from build123d import *

# Parameters (mm, degrees)
PROFILE_SKETCH_W         = 25
PROFILE_SKETCH_H         = 10.810660172
THICKNESS_EXTRUDE_DEPTH  = 2
FILLETS_R                = 6
CONNECTION_CHAMFER_SIZE  = 0.75
CONNECTION_CHAMFER_SIZE2 = 1.810660172


with BuildPart() as part:
    # Profile Sketch → Thickness Extrude (new body)
    with BuildSketch(Plane(origin=(0, 0, 0), x_dir=(1, 0, 0), z_dir=(0, 1, 0))):
        with Locations((12.5, 5.405330086)):
            Rectangle(PROFILE_SKETCH_W, PROFILE_SKETCH_H)
    extrude(amount=THICKNESS_EXTRUDE_DEPTH)

    # Fillets
    fillets_edges = [part.edges().sort_by_distance(p)[0] for p in [
        (0, 1, -10.810660172),
        (25, 1, -10.810660172),
    ]]
    fillet(fillets_edges, radius=FILLETS_R)

    # Connection Chamfer
    connection_chamfer_edges = [part.edges().sort_by_distance(p)[0] for p in [
        (12.5, 0, 0),
        (12.5, 2, 0),
    ]]
    connection_chamfer_side = [part.faces().sort_by_distance(p)[0] for p in [
        (12.5, 1, 0),
    ]]
    chamfer(connection_chamfer_edges, length=CONNECTION_CHAMFER_SIZE, length2=CONNECTION_CHAMFER_SIZE2, reference=connection_chamfer_side[0])


solid = part.part
Could you check a few things on this model? Use its own coordinates, in mm. Give positions to 0.01 mm unless a question says otherwise; leave off trailing zeros. Write each loop counter-clockwise with the first axis right and the second up, starting at its lowest first coordinate (ties: lowest second). Pieces come first, ordered by that corner, then holes. Notation, with made-up numbers: (-6, 70.25) -> (18, 70.25) arc R28 ccw to (18, 89.25) -> close; hole circle Ø7 at (66.25, 24.25). An arc over 180 degrees is marked (long way). Answer as a JSON object with one key per item and string values.
Q1. Suppose I cut it at A-A on x = 7.25. Write out the boundary of the cut face in (y, z), then the cut area to 3 significant figures.
Taken from the geometry:
{"outline": "(0, -10.81) -> (2, -10.81) -> (2, -1.81) -> (1.25, 0) -> (0.75, 0) -> (0, -1.81) -> close", "area": "20.3 mm²"}
Q2. We'd pull the mould along Z, two halves only. Please class faces 1 (the flat face through (25, 1, -3)), 2 (the flat face through (12.32, 0.37, -0.92)), 3 (the cylindrical face through (23.289, 1.014, -9.006)): released by +Z, released by -Z, zero draft, split by the parting line, or undercut.
Taken from the geometry:
{"face 1": "zero draft", "face 2": "released by +Z", "face 3": "released by -Z"}
Q3. Suppose I cut it at C-C on z = -8.75. Write out the boundary of the cut face in (x, y), then the cut area to 3 significant figures.
Taken from the geometry:
{"outline": "(1.47, 0) -> (23.53, 0) -> (23.53, 2) -> (1.47, 2) -> close", "area": "44.1 mm²"}
Q4. Will this pin go through, and if not, where does the flat tip stop? pin 1 Ø1 at (y, z) = (0.5, -5.5) entering from -X.
Taken from the geometry:
{"pin 1": "stops at x = 0"}
Q5. Please list where these lines run through material, in increasing order: L1, parallel to X at y = 1.85, z = -6.5; L2, parallel to Z at x = 6, y = 1.45; L3, parallel to X at y = 0.5, z = -7.
Taken from the geometry:
{"L1": "x = 0.24 to 24.76", "L2": "z = -10.81 to -0.48", "L3": "x = 0.41 to 24.59"}
Q6. Suppose I cut it at B-B on y = 1.5. Write out the boundary of the cut face in (x, z), then the cut area to 3 significant figures.
Taken from the geometry:
{"outline": "(0, -4.81) arc R6 ccw to (6, -10.81) -> (19, -10.81) arc R6 ccw to (25, -4.81) -> (25, -0.6) -> (0, -0.6) -> close", "area": "240 mm²"}
